Study the drawing (mm; zero at the part's minimum x, y, z) and answer. A direction names the side the tool comes from. Coordinates: 2 decimals unless noted, no trailing zeros. Loops run counter-clockwise (first coordinate to the right, second up) from the corner with the lowest first, then second, coordinate; pieces in that order, holes last. Notation, with made-up numbers: (31, 56) -> (36, 56) arc R29 cw to (36, 94) -> close; hole circle Ø5 at (44, 53). An arc over 180 degrees is marked (long way). Answer as a JSON object with one key per item and string values. Group by question number.
Q1. The part is cut by section C-C on y = 22.25. Write down the section's boundary in (x, z), and give its area (3 significant figures).
Q2. The part is cut by section D-D on z = 18. Write down the section's boundary in (x, y), and give its area (3 significant figures).
Q3. Each of these flat-tipped pins is pushed along its axis until it touches: P1, Ø10, axis at y = 18, z = 10.5, coming from the +X side; P2, Ø7, axis at x = 7.09, y = 13.5, coming from the +Z side; P3, Ø5, axis at x = 24.5, z = 17, coming from the -Y side; P4, Ø2, axis at y = 19, z = 7.5, coming from the +X side. Where does it stop, or does it pass through?
Q4. The part is cut by section A-A on x = 22.25. Write down the section's boundary in (y, z).
Q5. Determine the mould class of the marked faces 1, 2 and 3 for opening direction X: released by +X, released by -X, zero draft, split by the parting line, or undercut.
Q6. The part is cut by section B-B on y = 13.5. Write down the section's boundary in (x, z) (1 decimal).
Q7. Straight lines are drawn through the part: line 1 along X through (y, z) = (13.5, 12.7) (1 decimal); line 2 along Y through (x, z) = (22.25, 13.3); line 3 along Z through (x, y) = (25, 18). For each, find the intervals that lie inside material, in ascending order. Write a range as [from, to].
Q8. For the marked faces 4, 5 and 6, determine the directions among +Z, -Z, +X, -X, +Y, -Y from which every point of the face is accessible in a straight line to the end or side of a thin tool.
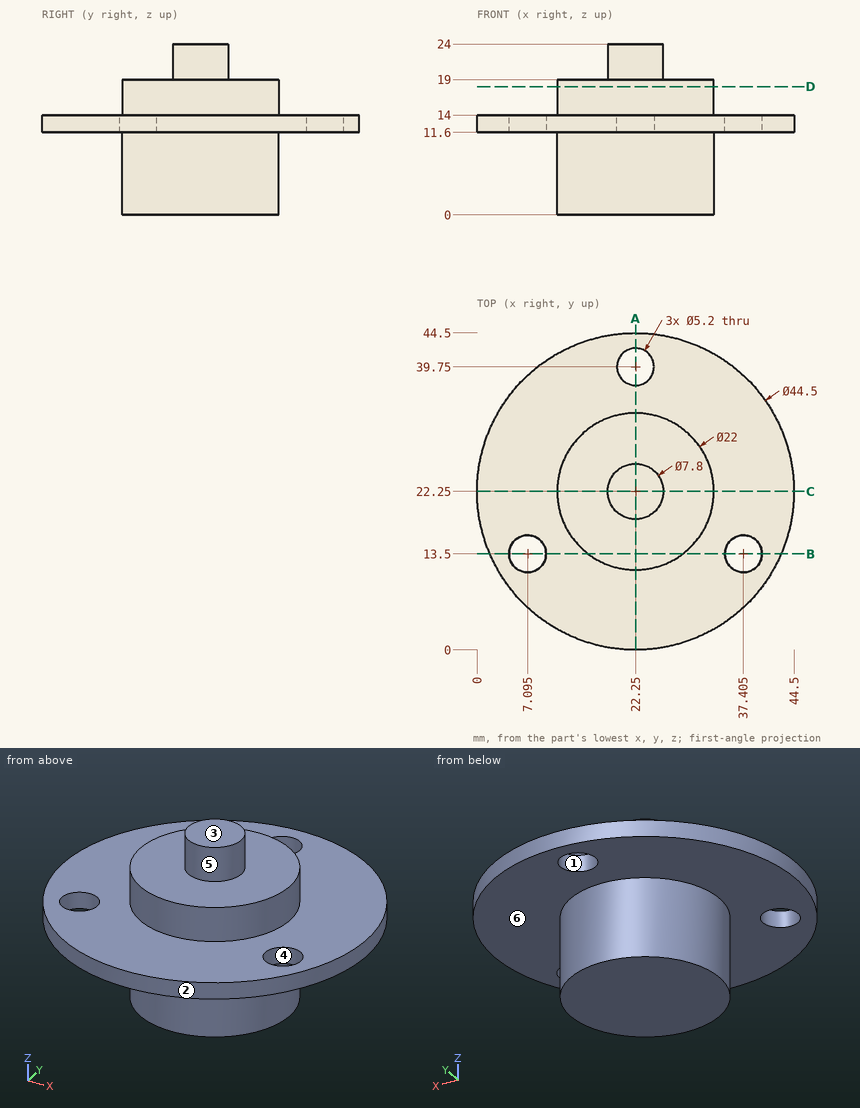
Final values:
{
 "1": {"outline": "(0, 11.6) -> (11.25, 11.6) -> (11.25, 0) -> (33.25, 0) -> (33.25, 11.6) -> (44.5, 11.6) -> (44.5, 14) -> (33.25, 14) -> (33.25, 19) -> (26.15, 19) -> (26.15, 24) -> (18.35, 24) -> (18.35, 19) -> (11.25, 19) -> (11.25, 14) -> (0, 14) -> close", "area": "511 mm2"},
 "2": {"outline": "circle Ø22 at (22.25, 22.25)", "area": "380 mm2"},
 "3": {"P1": "stops at x = 44.5", "P2": "stops at z = 14", "P3": "stops at y = 11.25", "P4": "stops at x = 33.02"},
 "4": {"outline": "(0, 11.6) -> (11.25, 11.6) -> (11.25, 0) -> (33.25, 0) -> (33.25, 11.6) -> (37.15, 11.6) -> (37.15, 14) -> (33.25, 14) -> (33.25, 19) -> (26.15, 19) -> (26.15, 24) -> (18.35, 24) -> (18.35, 19) -> (11.25, 19) -> (11.25, 14) -> (0, 14) -> close; (42.35, 11.6) -> (44.5, 11.6) -> (44.5, 14) -> (42.35, 14) -> close"},
 "5": {"face 1": "undercut", "face 2": "split by the parting line", "face 3": "zero draft"},
 "6": {"outline": "(1.8, 11.6) -> (4.5, 11.6) -> (4.5, 14) -> (1.8, 14) -> close; (9.7, 11.6) -> (15.6, 11.6) -> (15.6, 0) -> (28.9, 0) -> (28.9, 11.6) -> (34.8, 11.6) -> (34.8, 14) -> (28.9, 14) -> (28.9, 19) -> (15.6, 19) -> (15.6, 14) -> (9.7, 14) -> close; (40, 11.6) -> (42.7, 11.6) -> (42.7, 14) -> (40, 14) -> close"},
 "7": {"line 1": "x = [1.8, 4.5], [9.7, 34.8], [40, 42.7]", "line 2": "y = [0, 37.15], [42.35, 44.5]", "line 3": "z = [0, 19]"},
 "8": {"face 4": "+Z, -Z", "face 5": "+Z", "face 6": "-Z"}
}
